from build123d import *

# Parameters (mm, degrees)
SKETCH_1_R          = 5
EXTRUDE_1_DEPTH     = 7
M2_5X0_45_1_D       = 2.05
CUT_EXTRUDE_1_DEPTH = 0.8
CUT_EXTRUDE_3_DEPTH = 0.8


with BuildPart() as part:
    # 草图1 → 凸台-拉伸1 (new body)
    with BuildSketch(Plane.XY):
        Polygon((-15, 10), (-15, 16), (-27.5, 16), (-27.5, -16), (-15, -16), (-15, -10), (15, -10), (15, -16), (27.5, -16), (27.5, 16), (15, 16), (15, 10), align=None)
        Circle(SKETCH_1_R, mode=Mode.SUBTRACT)
    extrude(amount=EXTRUDE_1_DEPTH)

    # M2.5x0.45 螺纹孔1 (through all)
    with Locations(Plane(origin=(-20, 16, 3.5), x_dir=(0, 0, 1), z_dir=(0, 1, 0))):
        with Locations((0, 0), (0, 40)):
            Hole(M2_5X0_45_1_D / 2)

    # 草图4 → 切除-拉伸1 (cut, symmetric)
    with BuildSketch(Plane(origin=(0, 13, 0), x_dir=(1, 0, 0), z_dir=(0, 1, 0))):
        Polygon((-22, -4.654700538), (-22, -7), (-18, -7), (-18, -4.654700538), (-18, -2.345299462), (-20, -1.190598923), (-22, -2.345299462), align=None)
        Polygon((20, -1.190598923), (18, -2.345299462), (18, -4.654700538), (18, -7), (22, -7), (22, -4.654700538), (22, -2.345299462), align=None)
    extrude(amount=CUT_EXTRUDE_1_DEPTH, both=True, mode=Mode.SUBTRACT)

    # 草图7 → 切除-拉伸3 (cut, symmetric)
    with BuildSketch(Plane(origin=(0, -13, 0), x_dir=(-1, 0, 0), z_dir=(0, -1, 0))):
        Polygon((-22, -4.654700538), (-22, -7), (-18, -7), (-18, -4.654700538), (-18, -2.345299462), (-20, -1.190598923), (-22, -2.345299462), align=None)
        Polygon((20, -1.190598923), (18, -2.345299462), (18, -4.654700538), (18, -7), (22, -7), (22, -4.654700538), (22, -2.345299462), align=None)
    extrude(amount=CUT_EXTRUDE_3_DEPTH, both=True, mode=Mode.SUBTRACT)


solid = part.part
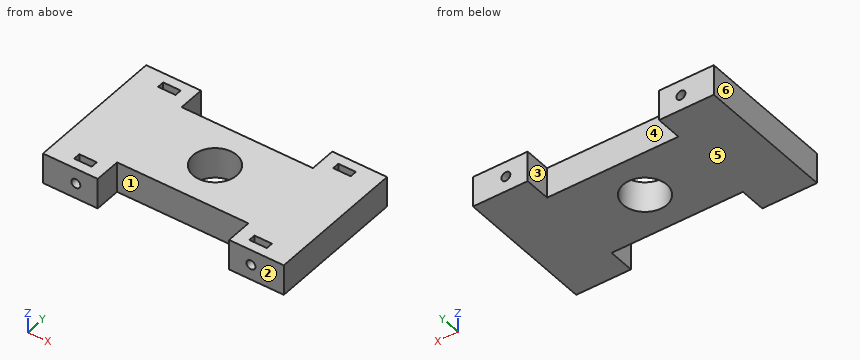
Input: part model. Units: mm. Frame: model coordinates. Face numbers are marked on the shaded views. A direction names the side the tool comes from. Coordinates: 2 decimals unless noted, no trailing zeros. Loops run counter-clockwise (first coordinate to the right, second up) from the corner with the lowest first, then second, coordinate; pieces in that order, holes last.
Q1. Cut plane A-A (y = 3). Output: boundary loops of the cut face in (x, z) (3 decimals).
Q2. Cut plane B-B (z = 6). Give the number of separate pieces and of enclosed holes in the cut face, then the cut area to 3 significant figures.
Q3. Draft query along X for the marked faces 3, 4, 5 and 6. Return one class per face: +X half, -X half, draft (parallel to the pull), parting line (faces both ways), or undercut.
Q4. Material intervals for line 1 (X direction, y = 14.8, z = 3.5) (3 decimals); line 2 (X direction, y = -12.5, z = 2.75); line 3 (Y direction, x = 0, z = 4.75), sorted ascending.
Q5. Set-up query: the marked faces 1 and 2. Return all of +Z, -Z, +X, -X, +Y, -Y with unobstructed straight access to the full face (end or side cutting, diameter ignored); none if empty.
Q6. Contact query for a flat-ended pin moving along its axis: pin 1 (2 mm diameter, centred on x = -2.5, z = 4, fed in from -Y). Output: stop coordinate, or through.
Q7. Cut plane D-D (x = -1.5). Output: boundary loops of the cut face in (y, z).
Working result:
1. outline: (-27.5, 0) - (-4, 0) - (-4, 7) - (-27.5, 7) - close; (4, 0) - (27.5, 0) - (27.5, 7) - (4, 7) - close; hole circle Ø2.05 at (-20, 3.5); hole circle Ø2.05 at (20, 3.5)
2. separate pieces: 1
2. enclosed holes: 5
2. area: 1,300 mm2
3. face 3: undercut
3. face 4: undercut
3. face 5: draft
3. face 6: -X half
4. line 1: x = -27.5 to -21.025, -18.975 to -15, 15 to 18.975, 21.025 to 27.5
4. line 2: x = -27.5 to -22, -18 to -15, 15 to 18, 22 to 27.5
4. line 3: y = -10 to -5, 5 to 10
5. face 1: +Z, -Z, -Y
5. face 2: +Z, -Z, +X, -X, -Y
6. pin 1: stops at y = -10
7. outline: (-10, 0) - (-4.77, 0) - (-4.77, 7) - (-10, 7) - close; (4.77, 0) - (10, 0) - (10, 7) - (4.77, 7) - close
